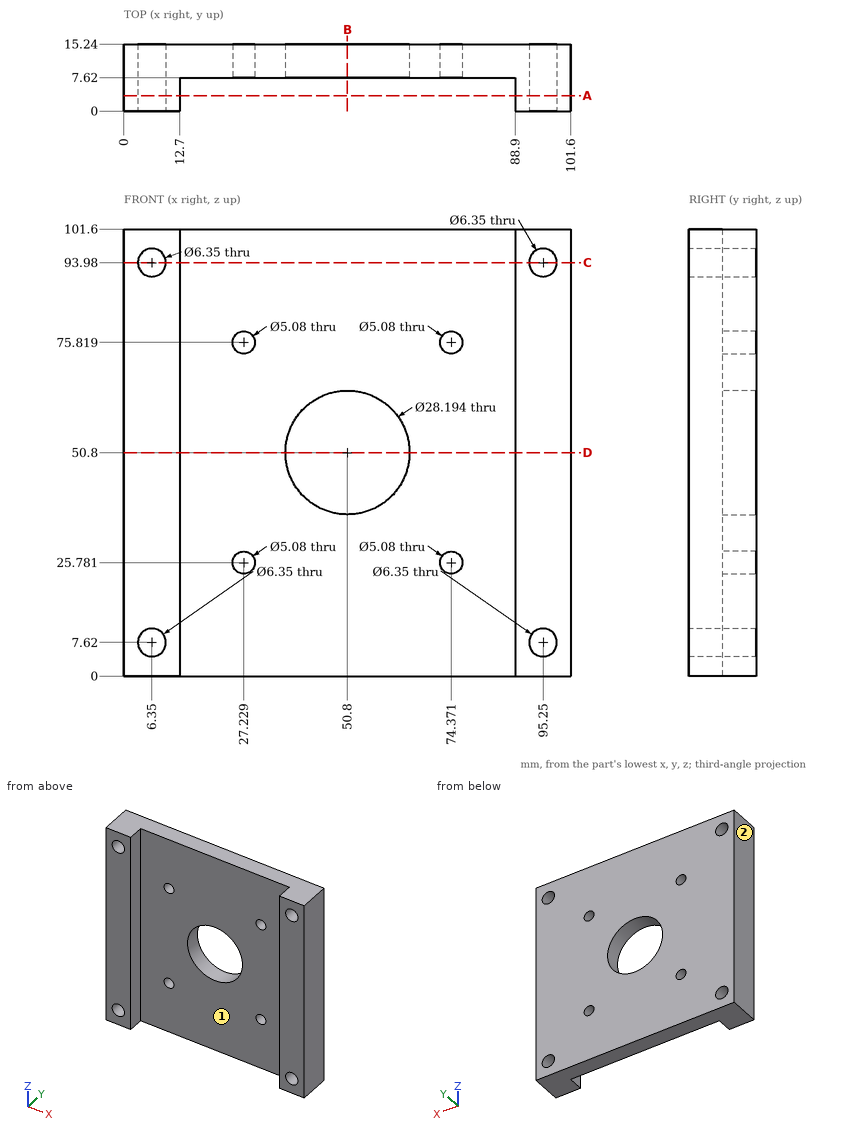
Geometry: see drawing. Coordinates: mm, zero at the bounding-box minimum. A direction names the side the tool comes from. Give positions to 0.01 mm unless a question says otherwise; leave off trailing zeros. Order: outer loops, then holes, each group sorted by start corner. A loop starts at its lowest first (then second) coordinate and runs counter-clockwise, first axis right, second up. Notation, with made-up numbers: (15.25, 20) - (64.25, 20) arc R9 ccw to (64.25, 32) - close; hole circle Ø10 at (46, -3). An arc over 180 degrees is marked (long way). One line per item, written item: value.
1. Cut plane A-A, the plane y = 3.5. Output: boundary loops of the cut face in (x, z) (3 decimals).
Determined:
outline: (0, 0) - (12.7, 0) - (12.7, 101.6) - (0, 101.6) - close; (88.9, 0) - (101.6, 0) - (101.6, 101.6) - (88.9, 101.6) - close; hole circle Ø6.35 at (6.35, 7.62); hole circle Ø6.35 at (6.35, 93.98); hole circle Ø6.35 at (95.25, 7.62); hole circle Ø6.35 at (95.25, 93.98)
2. Line query: probe 1 along X at (y, z) = (6, 7.62) (3 decimals); probe 2 along X at (y, z) = (4.5, 33); probe 3 along X at (y, z) = (11, 50.5). Output: solid intervals per line, ascending.
Determined:
probe 1: 0 to 3.175, 9.525 to 12.7, 88.9 to 92.075, 98.425 to 101.6
probe 2: 0 to 12.7, 88.9 to 101.6
probe 3: 0 to 36.71, 64.89 to 101.6
3. Cut plane C-C, the plane z = 93.98. Output: boundary loops of the cut face in (x, y) (3 decimals).
Determined:
outline: (0, 0) - (3.175, 0) - (3.175, 15.24) - (0, 15.24) - close; (9.525, 0) - (12.7, 0) - (12.7, 7.62) - (88.9, 7.62) - (88.9, 0) - (92.075, 0) - (92.075, 15.24) - (9.525, 15.24) - close; (98.425, 0) - (101.6, 0) - (101.6, 15.24) - (98.425, 15.24) - close
4. Pin query (flat end, axial travel): pin 1 Ø2 at (y, z) = (11, 36) entering from -X; pin 2 Ø4 at (x, z) = (27.23, 75.82) entering from +Y; pin 3 Ø6 at (x, z) = (74.37, 25.78) entering from -Y. Return the tip coordinate at first contact, or that it passes through.
Determined:
pin 1: x = 0
pin 2: through
pin 3: y = 7.62
5. Reachability of the marked faces 1 and 2 from +Z, -Z, +X, -X, +Y, -Y: full face, straight path, thin tool, end or side. Return the list, or none.
Determined:
face 1: +Z, -Z, -Y
face 2: +Z, -Z, -X, +Y, -Y
6. Cut plane B-B, the plane x = 50.8. Output: boundary loops of the cut face in (y, z), and give its area (3 significant figures).
Determined:
outline: (7.62, 0) - (15.24, 0) - (15.24, 36.7) - (7.62, 36.7) - close; (7.62, 64.9) - (15.24, 64.9) - (15.24, 101.6) - (7.62, 101.6) - close
area: 559 mm2
7. Cut plane D-D, the plane z = 50.8. Output: boundary loops of the cut face in (x, y).
Determined:
outline: (0, 0) - (12.7, 0) - (12.7, 7.62) - (36.7, 7.62) - (36.7, 15.24) - (0, 15.24) - close; (64.9, 7.62) - (88.9, 7.62) - (88.9, 0) - (101.6, 0) - (101.6, 15.24) - (64.9, 15.24) - close
